Source: CAD feature listing. Evaluate the final solid. Frame: model axes, mm. Face numbers are marked on the shaded views. Coordinates: 2 decimals unless noted, no trailing zeros. Loops run counter-clockwise (first coordinate to the right, second up) from the corner with the lowest first, then second, coordinate; pieces in that order, holes last. Notation, with made-up numbers: (84, -14) -> (103, -14) arc R31 ccw to (103, 10) -> close; hole circle Ø2 at (-32.75, 57). An arc over 180 degrees is marked (long way). Answer as a JSON object with one key per item and string values. Group by question number.
from build123d import *

# Parameters (mm, degrees)
BOX002_W               = 4
BOX002_H               = 4
BOX002_DEPTH           = 4
CYLINDER001_R          = 0.7
CYLINDER001_DEPTH      = 10
CYLINDER_R             = 0.7
CYLINDER_DEPTH         = 10
BOX001_W               = 1.25
BOX001_H               = 1.25
BOX001_DEPTH           = 2.5
BOX001_PLACEMENT_ANGLE = 45
BOX_W                  = 7.62
BOX_H                  = 7.62
BOX_DEPTH              = 2.5
CUT_PLACEMENT_ANGLE    = 90


with BuildPart() as lens_cut:
    # Box002 → Box002 (new body)
    with BuildSketch(Plane(origin=(-2, -2, -4), x_dir=(1, 0, 0), z_dir=(0, 0, 1))):
        with Locations((2, 2)):
            Rectangle(BOX002_W, BOX002_H)
    extrude(amount=BOX002_DEPTH)


with BuildPart() as led_lens001:
    # Sphere → Sphere (revolve)
    with BuildSketch(Plane.XZ):
        with BuildLine():
            ThreePointArc((0, -1.5), (1.5, 0), (0, 1.5))
            Line((0, 1.5), (0, -1.5))
        make_face()
    revolve(axis=Axis((0, 0, 0), (0, 0, 1)))

    # Cut003: cut Lens_cut
    add(lens_cut.part, mode=Mode.SUBTRACT)


with BuildPart() as led_lens001_1:
    # Cut003 placement: moved
    add(led_lens001.part.moved(Location((3.81, -3.81, 7.5))))


with BuildPart() as cut_led_right:
    # Cylinder001 → Cylinder001 (new body)
    with BuildSketch(Plane(origin=(3.81, -7.62, 0), x_dir=(1, 0, 0), z_dir=(0, 0, 1))):
        Circle(CYLINDER001_R)
    extrude(amount=CYLINDER001_DEPTH)


with BuildPart() as cut_led_left:
    # Cylinder → Cylinder (new body)
    with BuildSketch(Plane(origin=(3.81, 0, 0), x_dir=(1, 0, 0), z_dir=(0, 0, 1))):
        Circle(CYLINDER_R)
    extrude(amount=CYLINDER_DEPTH)


with BuildPart() as cut_cube:
    # Box001 → Box001 (new body)
    with BuildSketch(Plane.XY):
        with Locations((0.625, 0.625)):
            Rectangle(BOX001_W, BOX001_H)
    extrude(amount=BOX001_DEPTH)


with BuildPart() as cut_cube_1:
    # Box001 placement: moved
    add(cut_cube.part.moved(Location((7.62, 6.73612, 0))).rotate(Axis((7.62, 6.73612, 0), (0, 0, 1)), BOX001_PLACEMENT_ANGLE))


with BuildPart() as led_head002:
    # Box → Box (new body)
    with BuildSketch(Plane.XY):
        with Locations((3.81, 3.81)):
            Rectangle(BOX_W, BOX_H)
    extrude(amount=BOX_DEPTH)

    # Cut: cut cut_cube
    add(cut_cube_1.part, mode=Mode.SUBTRACT)


with BuildPart() as led_head002_1:
    # Cut placement: moved
    add(led_head002.part.moved(Location((7.62, -7.62, 5))).rotate(Axis((7.62, -7.62, 5), (0, 0, 1)), CUT_PLACEMENT_ANGLE))

    # Cut001: cut Cut_LED_left
    add(cut_led_left.part, mode=Mode.SUBTRACT)

    # Cut002: cut Cut_LED_right
    add(cut_led_right.part, mode=Mode.SUBTRACT)

    # Fusion008: union LED_lens001
    add(led_lens001_1.part)


with BuildPart() as led_head002_2:
    # Fusion008 placement: moved
    add(led_head002_1.part.moved(Location((-1.27, 1.27, -2.5))))


solid = led_head002_2.part
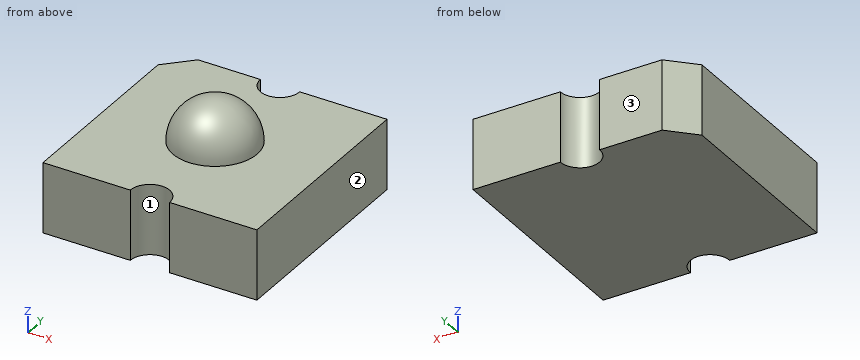
1. Pin query (flat end, axial travel): pin 1 Ø2 at (x, y) = (2, -0.5) entering from +Z; pin 2 Ø3 at (x, y) = (0, -0.5) entering from +Z. Return the tip coordinate at first contact, or that it passes through.
2. Section query A-A on z = 3.85. Return loops of the section in (x, y).
3. Section query C-C on y = -3. Return loops of the section in (x, z).
4. Section query B-B on x = 2.54. Return loops of the section in (y, z), then the cut area to 3 significant figures.
5. Section query D-D on y = -4.5. Return loops of the section in (x, z), then the cut area to 4 significant figures.
6. Ray query, L1, parallel to Z at x = 3.25, y = -6; L2, parallel to X at y = 0.75, z = 3.1; L3, parallel to Y at x = -0.5, z = 4.15. Return the intervals inside material, ascending.
7. Mould query, pull axis X, two halves, no side actions, for the marked faces 1, 2 and 3. Classes: pulls with the +X half, pulls with the -X half, needs draft (parallel to the pull), parting line crosses it, or undercut.
Solved:
{
 "1": {"pin 1": "z = 6.01", "pin 2": "z = 5"},
 "2": {"outline": "(-1.27, -6.35) -> (1.84, -6.35) arc R0.7 cw to (3.24, -6.35) -> (6.35, -6.35) -> (6.35, 1.27) -> (3.24, 1.27) arc R0.7 cw to (1.84, 1.27) -> (-0.39, 1.27) -> (-1.27, 0.39) -> close"},
 "3": {"outline": "(-1.27, 2.5) -> (6.35, 2.5) -> (6.35, 5) -> (3.97, 5) arc R1.43 ccw to (1.11, 5) -> (-1.27, 5) -> close"},
 "4": {"outline": "(-5.65, 2.5) -> (0.57, 2.5) -> (0.57, 5) -> (-1.04, 5) arc R1.5 ccw to (-4.04, 5) -> (-5.65, 5) -> close", "area": "19.1 mm^2"},
 "5": {"outline": "(-1.27, 2.5) -> (6.35, 2.5) -> (6.35, 5) -> (-1.27, 5) -> close", "area": "19.05 mm^2"},
 "6": {"L1": "2.5 to 5", "L2": "-0.91 to 2.07, 3.01 to 6.35", "L3": "-6.35 to 1.16"},
 "7": {"face 1": "undercut", "face 2": "pulls with the +X half", "face 3": "needs draft"}
}
